Can you work these out from the model? Positions are in its coordinate system, mm. Coordinates: 2 decimals unless noted, no trailing zeros. Loops run counter-clockwise (first coordinate to the right, second up) from the corner with the lowest first, then second, coordinate; pieces in that order, holes last. Notation, with made-up numbers: M -11.5,-29.75 L 12.5,-29.75 A16 ccw 12.5,-12.75 Z; hole C 15,21.5 d7. An arc over 180 degrees is marked long. Answer as a JSON object with one key per item and string values. Group by question number.
Item 1: Suppose I cut it at A-A (z = 5.5). Write out the boundary of the cut face in (x, y).
Item 2: If I drill on line 1 (Z direction, x = 0, y = 7.5); line 2 (X direction, y = 2.25, z = 5.5); line 3 (Z direction, x = -18, y = 7.25), over which ranges is the centre line in solid material (lowest first)?
Item 3: Suppose I cut it at D-D (z = -5.5). Write out the boundary of the cut face in (x, y), then the cut area to 3 significant figures.
Item 4: Suppose I cut it at C-C (x = -17.5). Write out the boundary of the cut face in (y, z), then the cut area to 3 significant figures.
Item 5: Suppose I cut it at B-B (y = 2.75). Write out the boundary of the cut face in (x, z).
Item 6: I'm going to push flat-ended pins straight in: pin 1 Ø2 at (x, y) = (4.5, 4.5) entering from +Z; pin 2 Ø1 at (x, y) = (4, 5.5) entering from -Z; pin 3 Ø3 at (x, y) = (-6.5, 5.5) entering from -Z. Where does each tip first touch, or does it pass through?
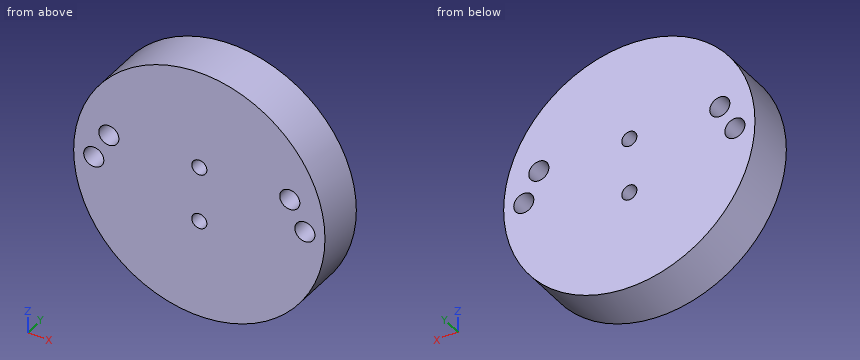
Autodesk Inventor part; units mm, degrees
ref_plane "YZ Plane" through (0, 0, 0) normal (1, 0, 0) x (0, 1, 0)
ref_plane "XZ Plane" through (0, 0, 0) normal (0, 1, 0) x (-1, 0, 0)
ref_plane "XY Plane" through (0, 0, 0) normal (0, 0, 1) x (1, 0, 0)
sketch "Sketch1" plane through (0, 0, 0) normal (0, 1, 0) x (-1, 0, 0)
  circle A0 centre (0, 0) radius 25
  dimension "d0" = 50
extrude "Extrusion1" add sketch "Sketch1" along normal blind 10
sketch "Sketch2" plane through (0, 10, 0) normal (0, 1, 0) x (1, 0, 0)
  circle A0 centre (0, -5.5) radius 1.5
  circle A1 centre (0, 5.5) radius 1.5
  circle A2 centre (-18, -5.5) radius 2
  circle A3 centre (-21, 0) radius 2
  circle A4 centre (21, 0) radius 2
  circle A5 centre (18, -5.5) radius 2
  point P0 (0, 0)
  dimension "d3" = 3
  dimension "d4" = 3
  dimension "d5" = 5.5
  dimension "d6" = 5.5
  dimension "d7" = 4
  dimension "d8" = 4
  dimension "d9" = 4
  dimension "d10" = 4
  dimension "d11" = 21
  dimension "d12" = 21
  dimension "d13" = 18
  dimension "d14" = 18
extrude "Extrusion2" cut sketch "Sketch2" against normal blind 10
properties part number "cABEZOTE"
From the geometry:
{
 "1": {"outline": "M -24.39,0 L -20,0 L -20,10 L -24.39,10 Z; M -16,0 L -1.5,0 L -1.5,10 L -16,10 Z; M 1.5,0 L 16,0 L 16,10 L 1.5,10 Z; M 20,0 L 24.39,0 L 24.39,10 L 20,10 Z"},
 "2": {"line 1": "-25 to -7, -4 to 4, 7 to 25", "line 2": "-24.39 to -20, -16 to -1.5, 1.5 to 16, 20 to 24.39", "line 3": "-17.35 to 3.5, 7.5 to 17.35"},
 "3": {"outline": "M -24.39,0 L -1.5,0 L -1.5,10 L -24.39,10 Z; M 1.5,0 L 24.39,0 L 24.39,10 L 1.5,10 Z", "area": "458 mm2"},
 "4": {"outline": "M 0,-17.85 L 10,-17.85 L 10,3.56 L 0,3.56 Z; M 0,7.44 L 10,7.44 L 10,17.85 L 0,17.85 Z", "area": "318 mm2"},
 "5": {"outline": "C 0,0 d50; hole C -21,0 d4; hole C -18,5.5 d4; hole C 0,-5.5 d3; hole C 0,5.5 d3; hole C 18,5.5 d4; hole C 21,0 d4"},
 "6": {"pin 1": "z = 24.75", "pin 2": "z = -24.75", "pin 3": "z = -24.49"}
}
